Here's how the part is built. I have some questions about the finished solid (model axes, mm). A direction names the side the tool comes from. Round coordinates to 2 decimals unless told otherwise and drop trailing zeros. Write each loop counter-clockwise with the first axis right and the second up, starting at its lowest first coordinate (ties: lowest second). Pieces come first, ordered by that corner, then holes. Notation, with made-up numbers: M 66.5,55.25 L 125.5,55.25 A26 cw 125.5,85.25 Z; hole C -31,22.25 d6. An arc over 180 degrees is marked long. Use one line per item in the form item = value. Start each with the question number.
Q1. I want a section at A-A on y = 10. List the corners of the cut face in (x, z) for me.
Q2. I want a section at B-B on z = -20. List the corners of the cut face in (x, y) for me.
Q3. I want a section at D-D on z = -2. List the corners of the cut face in (x, y) for me, and give its area (3 significant figures).
Q4. I'm going to push flat-ended pins straight in: pin 1 Ø1.2 at (y, z) = (24, 2) entering from -X; pin 2 Ø13 at (x, z) = (-9, 1) entering from +Y. Where does each tip first touch, or does it pass through?
Q5. We'd pull the mould along Z, two halves only. Please class faces 1 (the face through (-1, 13, 25)), 2 (the face through (-1, 0, 0)), 3 (the face through (34.5, 13, 0)): +Z half, -Z half, draft (parallel to the pull), parting line (faces both ways), or undercut.
Q6. I want a section at C-C on x = 16. List the corners of the cut face in (y, z) for me, and give its area (3 significant figures).
Q7. I need wall thicknesses on line 1 along Z through (x, y) = (17, 19); line 2 along X through (y, z) = (6, 2); line 3 along Z through (x, y) = (8, 24.25). Which ranges of each line are inside material? Lowest first, please. Write a range as from..to.
Q8. For faces 4 (the face through (-12, 23.04, -23)), 5 (the face through (34.5, 25, 0)), 6 (the face through (0, 3, 0)), which set-ups out of +Z, -Z, +X, -X, +Y, -Y let a thin tool reach every point of the face, with its end or its side?
```python
from build123d import *

# Parameters (mm, degrees)
CROQUIS1_W              = 75
CROQUIS1_H              = 50
CROQUIS1_W_2            = 69
CROQUIS1_H_2            = 44
SALIENTE_EXTRUIR1_DEPTH = 26
CROQUIS1_2_W            = 69
CROQUIS1_2_H            = 44
SALIENTE_EXTRUIR2_DEPTH = 3
CROQUIS3_W              = 1.48
CROQUIS3_H              = 1.48
CORTAR_EXTRUIR1_DEPTH   = 72
CROQUIS4_W              = 46.96
CROQUIS4_H              = 1.48
CORTAR_EXTRUIR2_DEPTH   = 1.5
CROQUIS7_W              = 1.5
CROQUIS7_H              = 7
CORTAR_EXTRUIR3_DEPTH   = 0.32


with BuildPart() as part:
    # Croquis1 → Saliente-Extruir1 (new body)
    with BuildSketch(Plane(origin=(0, 0, 0), x_dir=(1, 0, 0), z_dir=(0, 1, 0))):
        Rectangle(CROQUIS1_W, CROQUIS1_H)
        Rectangle(CROQUIS1_W_2, CROQUIS1_H_2, mode=Mode.SUBTRACT)
    extrude(amount=SALIENTE_EXTRUIR1_DEPTH)

    # Croquis1_2 → Saliente-Extruir2 (add)
    with BuildSketch(Plane(origin=(0, 0, 0), x_dir=(1, 0, 0), z_dir=(0, 1, 0))):
        Rectangle(CROQUIS1_2_W, CROQUIS1_2_H)
    extrude(amount=SALIENTE_EXTRUIR2_DEPTH)

    # Croquis3 → Cortar-Extruir1 (cut)
    with BuildSketch(Plane.ZY.offset(37.5)):
        Polygon((22, 26), (-22, 26), (-22, 24.52), (-22, 23.04), (22, 23.04), (22, 24.52), align=None)
        with Locations((-22.74, 23.78)):
            Rectangle(CROQUIS3_W, CROQUIS3_H)
        with Locations((22.74, 23.78)):
            Rectangle(CROQUIS3_W, CROQUIS3_H)
    extrude(amount=-CORTAR_EXTRUIR1_DEPTH, mode=Mode.SUBTRACT)

    # Croquis4 → Cortar-Extruir2 (cut)
    with BuildSketch(Plane.ZY.offset(-34.5)):
        with Locations((0, 23.78)):
            Rectangle(CROQUIS4_W, CROQUIS4_H)
    extrude(amount=-CORTAR_EXTRUIR2_DEPTH, mode=Mode.SUBTRACT)

    # Croquis7 → Cortar-Extruir3 (cut)
    with BuildSketch(Plane(origin=(0, 23.04, 0), x_dir=(1, 0, 0), z_dir=(0, 1, 0))):
        with Locations((-36.12, 0)):
            Rectangle(CROQUIS7_W, CROQUIS7_H)
    extrude(amount=-CORTAR_EXTRUIR3_DEPTH, mode=Mode.SUBTRACT)


solid = part.part
```
Reported:
q1.outline = M -37.5,-25 L 37.5,-25 L 37.5,25 L -37.5,25 Z; hole M -34.5,-22 L 34.5,-22 L 34.5,22 L -34.5,22 Z
q2.outline = M -37.5,0 L 37.5,0 L 37.5,26 L 34.5,26 L 34.5,24.52 L 36,24.52 L 36,23.04 L 34.5,23.04 L 34.5,3 L -34.5,3 L -34.5,23.04 L -37.5,23.04 Z
q3.outline = M -37.5,0 L 37.5,0 L 37.5,26 L 34.5,26 L 34.5,24.52 L 36,24.52 L 36,23.04 L 34.5,23.04 L 34.5,3 L -34.5,3 L -34.5,23.04 L -35.37,23.04 L -35.37,22.72 L -36.87,22.72 L -36.87,23.04 L -37.5,23.04 Z
q3.area = 351 mm^2
q4.pin_1 = 34.5
q4.pin_2 = 3
q5.face_1 = +Z half
q5.face_2 = draft
q5.face_3 = undercut
q6.outline = M 0,-25 L 26,-25 L 26,-22 L 24.52,-22 L 24.52,-23.48 L 23.04,-23.48 L 23.04,-22 L 3,-22 L 3,22 L 23.04,22 L 23.04,23.48 L 24.52,23.48 L 24.52,22 L 26,22 L 26,25 L 0,25 Z
q6.area = 284 mm^2
q7.line_1 = -25..-22, 22..25
q7.line_2 = -37.5..-34.5, 34.5..37.5
q7.line_3 = -25..-23.48, 23.48..25
q8.face_4 = -X
q8.face_5 = -X, +Y
q8.face_6 = +Y
